Build history of the part. All positions in model axes, mm. A direction names the side the tool comes from. Give positions to 0.01 mm unless a question says otherwise; leave off trailing zeros. Write each loop counter-clockwise with the first axis right and the second up, starting at its lowest first coordinate (ties: lowest second). Pieces come first, ordered by that corner, then holes. Notation, with made-up numbers: M 38,-7 L 85,-7 A14 ccw 85,15 Z; hole C -9,53 d7. An arc over 180 degrees is marked long. Return JSON: item names as keys, results as strings. Group by question number.
Q1. Band-saw the part on B-B, the plane y = 34. Give the cut face in (x, z) (3 decimals).
Q2. Band-saw the part on A-A, the plane z = 5.25. Give the cut face in (x, y) (3 decimals).
Q3. Wall check: probe 1 along X at (y, z) = (24, -5) (3 decimals); probe 2 along X at (y, z) = (59, 9.25); probe 3 along Z at (x, y) = (6.5, 61) (3 decimals). Give the ranges that are in metal, low to high.
Q4. Flat gauge pins, fed straight in: pin 1 Ø1.1 at (x, z) = (57.5, -4.5) entering from +Y; pin 2 Ø19.5 at (x, y) = (33, 35) entering from +Z (3 decimals); pin 3 Ø2 at (y, z) = (9.5, -7) entering from +X. Where does each tip first touch, or does it go through?
Q5. Band-saw the part on C-C, the plane x = 14.5. Give the cut face in (y, z) (3 decimals), then the cut area to 3 significant figures.
Q6. Pull direction Z, two halves, no side cores. Call faces 1 (the cylindrical face through (5.565, 5.696, -0.098)), 2 (the flat face through (71.12, 43, 0)), 3 (the flat face through (67.945, 44, 0)), 4 (the flat face through (5, 39, 10.16)): +Z half, -Z half, draft (parallel to the pull), parting line (faces both ways), or undercut.
Q7. Band-saw the part on D-D, the plane z = -5.75. Give the cut face in (x, y) (3 decimals).
Q8. Tool access for faces 5 (the flat face through (7, 40, 6.985)), 6 (the flat face through (58, 3.175, -6)), 7 (the flat face through (61.087, 36, 8)), 8 (the flat face through (35, 76.2, -8)), 9 (the flat face through (35, 39, -10.16)): list every direction of +Z, -Z, +X, -X, +Y, -Y with a clear straight run to the whole face (end or side of a thin tool).
from build123d import *

# Parameters (mm, degrees)
SKETCH1_W           = 71.12
SKETCH1_H           = 76.2
BOSS_EXTRUDE1_DEPTH = 10.16
SKETCH2_W           = 64.77
SKETCH2_H           = 13.97
CUT_EXTRUDE1_DEPTH  = 73.025
SKETCH10_W          = 51.054
SKETCH10_H          = 17.145
CUT_EXTRUDE2_DEPTH  = 77.2
FILLET5_R           = 8.382
FILLET3_R           = 8.382
CUT_EXTRUDE3_DEPTH  = 21.32


with BuildPart() as part:
    # Sketch1 → Boss-Extrude1 (new body, symmetric)
    with BuildSketch(Plane.XY):
        with Locations((35.56, 38.1)):
            Rectangle(SKETCH1_W, SKETCH1_H)
    extrude(amount=BOSS_EXTRUDE1_DEPTH, both=True)

    # Sketch2 → Cut-Extrude1 (cut)
    with BuildSketch(Plane(origin=(0, 76.2, 0), x_dir=(1, 0, 0), z_dir=(0, 1, 0))):
        with Locations((35.56, 0)):
            Rectangle(SKETCH2_W, SKETCH2_H)
    extrude(amount=-CUT_EXTRUDE1_DEPTH, mode=Mode.SUBTRACT)

    # Sketch10 → Cut-Extrude2 (cut, through all)
    with BuildSketch(Plane(origin=(0, 76.2, 0), x_dir=(1, 0, 0), z_dir=(0, 1, 0))):
        with Locations((35.56, -1.5875)):
            Rectangle(SKETCH10_W, SKETCH10_H)
    extrude(amount=-CUT_EXTRUDE2_DEPTH, mode=Mode.SUBTRACT)

    # Fillet5
    fillet5_edges = [part.edges().sort_by_distance(p)[0] for p in [
        (61.087, 1.5875, -6.985),
        (10.033, 1.5875, -6.985),
    ]]
    fillet(fillet5_edges, radius=FILLET5_R)

    # Fillet3
    fillet3_edges = [part.edges().sort_by_distance(p)[0] for p in [
        (67.945, 3.175, 0),
        (3.175, 3.175, 0),
    ]]
    fillet(fillet3_edges, radius=FILLET3_R)

    # Sketch11 → Cut-Extrude3 (cut, through all)
    with BuildSketch(Plane.XY.offset(10.16)):
        with BuildLine():
            Line((0, 11.557), (0, 0))
            Line((0, 0), (11.557, 0))
            ThreePointArc((11.557, 0), (3.38496693, 3.38496693), (0, 11.557))
        make_face()
        with BuildLine():
            Line((71.12, 11.557), (71.12, 0))
            Line((71.12, 0), (59.563, 0))
            ThreePointArc((59.563, 0), (67.73503307, 3.38496693), (71.12, 11.557))
        make_face()
    extrude(amount=-CUT_EXTRUDE3_DEPTH, mode=Mode.SUBTRACT)


solid = part.part
From the geometry:
{
 "1": {"outline": "M 0,-10.16 L 71.12,-10.16 L 71.12,10.16 L 61.087,10.16 L 61.087,6.985 L 67.945,6.985 L 67.945,-6.985 L 3.175,-6.985 L 3.175,6.985 L 10.033,6.985 L 10.033,10.16 L 0,10.16 Z"},
 "2": {"outline": "M 0,11.557 A11.557 ccw 10.033,0.101 L 10.033,3.315 A8.382 cw 3.175,11.557 L 3.175,76.2 L 0,76.2 Z; M 61.087,0.101 A11.557 ccw 71.12,11.557 L 71.12,76.2 L 67.945,76.2 L 67.945,11.557 A8.382 cw 61.087,3.315 Z"},
 "3": {"probe 1": "x = 0 to 3.175, 67.945 to 71.12", "probe 2": "x = 0 to 10.03, 61.09 to 71.12", "probe 3": "z = -10.16 to -6.985, 6.985 to 10.16"},
 "4": {"pin 1": "passes through", "pin 2": "stops at z = -6.985", "pin 3": "stops at x = 71.07"},
 "5": {"outline": "M 0,-10.16 L 76.2,-10.16 L 76.2,-6.985 L 3.175,-6.985 L 3.175,-6.015 L 0,-6.015 Z", "area": "245 mm^2"},
 "6": {"face 1": "undercut", "face 2": "draft", "face 3": "undercut", "face 4": "+Z half"},
 "7": {"outline": "M 0,11.557 A11.557 ccw 11.557,0 L 14.036,0 L 14.036,3.175 L 11.557,3.175 A8.382 cw 3.175,11.557 L 3.175,76.2 L 0,76.2 Z; M 57.084,0 L 59.563,0 A11.557 ccw 71.12,11.557 L 71.12,76.2 L 67.945,76.2 L 67.945,11.557 A8.382 cw 59.563,3.175 L 57.084,3.175 Z"},
 "8": {"face 5": "+Y", "face 6": "+Z, +Y", "face 7": "+Z, +Y, -Y", "face 8": "+Z, -Z, +X, -X, +Y", "face 9": "-Z, +X, -X, +Y, -Y"}
}
